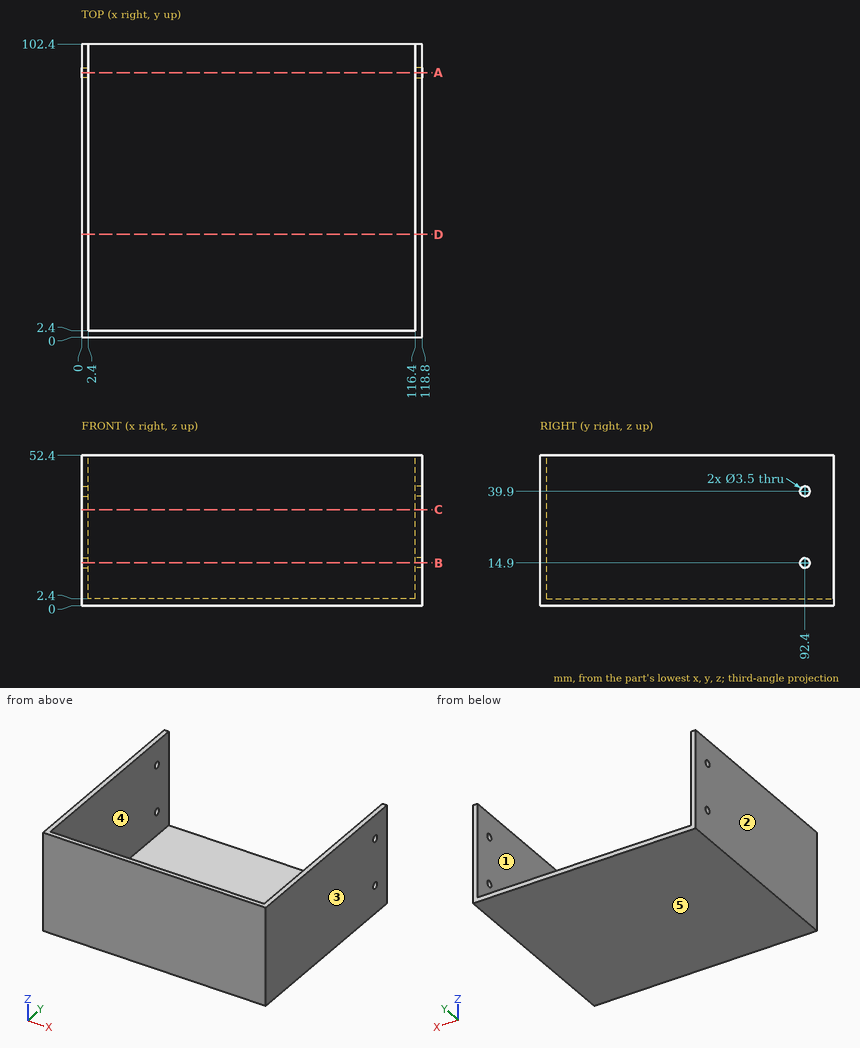
For this review, use the dimensioned drawing (mm, ordinates from the lowest corner) and the shaded views. A direction names the side the tool comes from. Round coordinates to 2 decimals unless told otherwise and drop trailing zeros. Order: outer loops, then holes, each group sorted by start corner. A loop starts at its lowest first (then second) coordinate and runs counter-clockwise, first axis right, second up.
1) Consider section B-B (z = 14.9). State the section outline as (x, y) points, plus the area to 3 significant figures.
The answers:
outline: (0, 0) - (118.8, 0) - (118.8, 90.65) - (116.4, 90.65) - (116.4, 2.4) - (2.4, 2.4) - (2.4, 90.65) - (0, 90.65) - close; (0, 94.15) - (2.4, 94.15) - (2.4, 102.4) - (0, 102.4) - close; (116.4, 94.15) - (118.8, 94.15) - (118.8, 102.4) - (116.4, 102.4) - close
area: 748 mm2
2) Draft analysis for pull direction X (two halves, no side actions). For the marked faces 3, 4 and 5, state which applies: released by +X, released by -X, zero draft, split by the parting line, or undercut.
The answers:
face 3: released by +X
face 4: undercut
face 5: zero draft
3) Consider section A-A (y = 92.4). State the section outline as (x, z) points.
The answers:
outline: (0, 0) - (118.8, 0) - (118.8, 13.15) - (116.4, 13.15) - (116.4, 2.4) - (2.4, 2.4) - (2.4, 13.15) - (0, 13.15) - close; (0, 16.65) - (2.4, 16.65) - (2.4, 38.15) - (0, 38.15) - close; (0, 41.65) - (2.4, 41.65) - (2.4, 52.4) - (0, 52.4) - close; (116.4, 16.65) - (118.8, 16.65) - (118.8, 38.15) - (116.4, 38.15) - close; (116.4, 41.65) - (118.8, 41.65) - (118.8, 52.4) - (116.4, 52.4) - close
4) Machinability: for the marked faces 1 and 2, which of the approach directions +Z, -Z, +X, -X, +Y, -Y give a long, thin tool a straight path to every point of the face, cutting with its end or side? Answer none if there is none.
The answers:
face 1: +Z, +Y
face 2: +Z, -Z, -X, +Y, -Y
5) Consider section C-C (z = 33.5). State the section outline as (x, y) points, plus the area to 3 significant figures.
The answers:
outline: (0, 0) - (118.8, 0) - (118.8, 102.4) - (116.4, 102.4) - (116.4, 2.4) - (2.4, 2.4) - (2.4, 102.4) - (0, 102.4) - close
area: 765 mm2
6) For L1, parallel to Z at x = 1.55, y = 92.4; L2, parallel to X at y = 38, z = 4; L3, parallel to Y at x = 44.5, z = 38.5, list the stretches that pass through material, from the lowest coordinate up.
The answers:
L1: z = 0 to 13.15, 16.65 to 38.15, 41.65 to 52.4
L2: x = 0 to 2.4, 116.4 to 118.8
L3: y = 0 to 2.4
7) Clearance check with flat-ended pins moving along their axes: pin 1 Ø15 at (x, z) = (75.5, 27) entering from +Y; pin 2 Ø3 at (y, z) = (92.4, 39.9) entering from -X; pin 3 Ø10 at (x, y) = (53.5, 25) entering from -Z. State where each tip first meets the part, or that it passes through.
The answers:
pin 1: stops at y = 2.4
pin 2: passes through
pin 3: stops at z = 0
8) Consider section D-D (y = 36). State the section outline as (x, z) points, plus the area to 3 significant figures.
The answers:
outline: (0, 0) - (118.8, 0) - (118.8, 52.4) - (116.4, 52.4) - (116.4, 2.4) - (2.4, 2.4) - (2.4, 52.4) - (0, 52.4) - close
area: 525 mm2
